from build123d import *

# Parameters (mm, degrees)
F1_DEPTH = 7.5


with BuildPart() as f1:
    # F0 (on Top) → F1 (new body)
    with BuildSketch(Plane.XY):
        with BuildLine():
            ThreePointArc((8.7951269587, 32.985141357), (9.3550716579, 31.5299513828), (9.8501945992, 30.0514490323))
            ThreePointArc((9.8501945992, 30.0514490323), (12.9209659931, 34.6103211779), (14, 40))
            ThreePointArc((14, 40), (-5.3896788221, 52.9209659931), (-9.8501945992, 30.0514490323))
            ThreePointArc((-9.8501945992, 30.0514490323), (-9.3550716579, 31.5299513828), (-8.7951269587, 32.985141357))
            ThreePointArc((-8.7951269587, 32.985141357), (-3.7160006536, 50.6185610674), (11.25, 40))
            ThreePointArc((11.25, 40), (10.6185610674, 36.2839993464), (8.7951269587, 32.985141357))
        make_face()
        with BuildLine():
            ThreePointArc((0, 26), (5.3254242297, 27.0524188833), (9.8501945992, 30.0514490323))
            ThreePointArc((9.8501945992, 30.0514490323), (9.3550716579, 31.5299513828), (8.7951269587, 32.985141357))
            ThreePointArc((8.7951269587, 32.985141357), (4.8808472762, 29.8639342017), (0, 28.75))
            Line((0, 28.75), (0, 26))
        make_face()
        with BuildLine():
            ThreePointArc((-9.8501945992, 30.0514490323), (-5.3254242297, 27.0524188833), (0, 26))
            Line((0, 26), (0, 28.75))
            ThreePointArc((0, 28.75), (-4.8808472762, 29.8639342017), (-8.7951269587, 32.985141357))
            ThreePointArc((-8.7951269587, 32.985141357), (-9.3550716579, 31.5299513828), (-9.8501945992, 30.0514490323))
        make_face()
        with BuildLine():
            ThreePointArc((0, 14), (5.4503386544, 12.8954956691), (10.040688359, 9.7562583646))
            ThreePointArc((10.040688359, 9.7562583646), (11.4358727735, 19.9178431142), (9.8501945992, 30.0514490323))
            ThreePointArc((9.8501945992, 30.0514490323), (5.3254242297, 27.0524188833), (0, 26))
            Line((0, 26), (0, 22.6483326405))
            Line((0, 22.6483326405), (5.2916659042, 22.6483326405))
            Line((5.2916659042, 22.6483326405), (5.2916659042, 14.8166660219))
            Line((5.2916659042, 14.8166660219), (0, 14.8166660219))
            Line((0, 14.8166660219), (0, 14))
        make_face()
        with BuildLine():
            ThreePointArc((-10.040688359, 9.7562583646), (-5.4503386544, 12.8954956691), (0, 14))
            Line((0, 14), (0, 14.8166660219))
            Line((0, 14.8166660219), (-5.7150004432, 14.8166660219))
            Line((-5.7150004432, 14.8166660219), (-5.7150004432, 22.6483326405))
            Line((-5.7150004432, 22.6483326405), (0, 22.6483326405))
            Line((0, 22.6483326405), (0, 26))
            ThreePointArc((0, 26), (-5.3254242297, 27.0524188833), (-9.8501945992, 30.0514490323))
            ThreePointArc((-9.8501945992, 30.0514490323), (-11.4358727735, 19.9178431142), (-10.040688359, 9.7562583646))
        make_face()
        with BuildLine():
            ThreePointArc((0, 11.25), (5.0410157742, 10.0573684413), (9.013218304, 6.7323395492))
            ThreePointArc((9.0132183039, 6.7323395492), (9.5611769089, 8.2326704367), (10.040688359, 9.7562583646))
            ThreePointArc((10.040688359, 9.7562583646), (5.4503386544, 12.8954956691), (0, 14))
            Line((0, 14), (0, 11.25))
        make_face()
        with BuildLine():
            ThreePointArc((9.013218304, 6.7323395492), (10.6761698638, 3.5470969877), (11.25, 0))
            Line((11.25, 0), (14, 0))
            ThreePointArc((14, 0), (12.9724638567, 5.2645210121), (10.040688359, 9.7562583646))
            ThreePointArc((10.040688359, 9.7562583646), (9.5611769089, 8.2326704367), (9.0132183039, 6.7323395492))
        make_face()
        with BuildLine():
            ThreePointArc((-9.013218304, 6.7323395492), (-5.0410157742, 10.0573684413), (0, 11.25))
            Line((0, 11.25), (0, 14))
            ThreePointArc((0, 14), (-5.4503386544, 12.8954956691), (-10.040688359, 9.7562583646))
            ThreePointArc((-10.040688359, 9.7562583646), (-9.5611769089, 8.2326704367), (-9.0132183039, 6.7323395492))
        make_face()
        with BuildLine():
            ThreePointArc((-11.25, 0), (-10.6761698638, 3.5470969877), (-9.013218304, 6.7323395492))
            ThreePointArc((-9.0132183039, 6.7323395492), (-9.5611769089, 8.2326704367), (-10.040688359, 9.7562583646))
            ThreePointArc((-10.040688359, 9.7562583646), (-12.9724638567, 5.2645210121), (-14, 0))
            Line((-14, 0), (-11.25, 0))
        make_face()
        with BuildLine():
            ThreePointArc((-10.040688359, -9.7562583646), (-9.5611769089, -8.2326704367), (-9.0132183039, -6.7323395492))
            ThreePointArc((-9.013218304, -6.7323395492), (-10.6761698638, -3.5470969877), (-11.25, 0))
            Line((-11.25, 0), (-14, 0))
            ThreePointArc((-14, 0), (-12.9724638567, -5.2645210121), (-10.040688359, -9.7562583646))
        make_face()
        with BuildLine():
            Line((14, 0), (11.25, 0))
            ThreePointArc((11.25, 0), (10.6761698638, -3.5470969877), (9.013218304, -6.7323395492))
            ThreePointArc((9.0132183039, -6.7323395492), (9.5611769089, -8.2326704367), (10.040688359, -9.7562583646))
            ThreePointArc((10.040688359, -9.7562583646), (12.9724638567, -5.2645210121), (14, 0))
        make_face()
        with BuildLine():
            ThreePointArc((10.040688359, -9.7562583646), (9.5611769089, -8.2326704367), (9.0132183039, -6.7323395492))
            ThreePointArc((9.013218304, -6.7323395492), (5.0410157742, -10.0573684413), (0, -11.25))
            Line((0, -11.25), (0, -14))
            ThreePointArc((0, -14), (5.4503386544, -12.8954956691), (10.040688359, -9.7562583646))
        make_face()
        with BuildLine():
            Line((0, -14), (0, -11.25))
            ThreePointArc((0, -11.25), (-5.0410157742, -10.0573684413), (-9.013218304, -6.7323395492))
            ThreePointArc((-9.0132183039, -6.7323395492), (-9.5611769089, -8.2326704367), (-10.040688359, -9.7562583646))
            ThreePointArc((-10.040688359, -9.7562583646), (-5.4503386544, -12.8954956691), (0, -14))
        make_face()
        with BuildLine():
            Line((0, -14.8166660219), (0, -14))
            ThreePointArc((0, -14), (-5.4503386544, -12.8954956691), (-10.040688359, -9.7562583646))
            ThreePointArc((-10.040688359, -9.7562583646), (-11.4358727735, -19.9178431142), (-9.8501945992, -30.0514490323))
            ThreePointArc((-9.8501945992, -30.0514490323), (-5.3254242297, -27.0524188833), (0, -26))
            Line((0, -26), (0, -22.6483326405))
            Line((0, -22.6483326405), (-5.7150004432, -22.6483326405))
            Line((-5.7150004432, -22.6483326405), (-5.7150004432, -14.8166660219))
            Line((-5.7150004432, -14.8166660219), (0, -14.8166660219))
        make_face()
        with BuildLine():
            ThreePointArc((9.8501945992, -30.0514490323), (11.4358727735, -19.9178431142), (10.040688359, -9.7562583646))
            ThreePointArc((10.040688359, -9.7562583646), (5.4503386544, -12.8954956691), (0, -14))
            Line((0, -14), (0, -14.8166660219))
            Line((0, -14.8166660219), (5.2916659042, -14.8166660219))
            Line((5.2916659042, -14.8166660219), (5.2916659042, -22.6483326405))
            Line((5.2916659042, -22.6483326405), (0, -22.6483326405))
            Line((0, -22.6483326405), (0, -26))
            ThreePointArc((0, -26), (5.3254242297, -27.0524188833), (9.8501945992, -30.0514490323))
        make_face()
        with BuildLine():
            ThreePointArc((14, -40), (12.9209659931, -34.6103211779), (9.8501945992, -30.0514490323))
            ThreePointArc((9.8501945992, -30.0514490323), (9.3550716579, -31.5299513828), (8.7951269587, -32.985141357))
            ThreePointArc((8.7951269587, -32.985141357), (10.6185610674, -36.2839993464), (11.25, -40))
            ThreePointArc((11.25, -40), (-3.7160006536, -50.6185610674), (-8.7951269587, -32.985141357))
            ThreePointArc((-8.7951269587, -32.985141357), (-9.3550716579, -31.5299513828), (-9.8501945992, -30.0514490323))
            ThreePointArc((-9.8501945992, -30.0514490323), (-5.3896788221, -52.9209659931), (14, -40))
        make_face()
        with BuildLine():
            Line((0, -28.75), (0, -26))
            ThreePointArc((0, -26), (-5.3254242297, -27.0524188833), (-9.8501945992, -30.0514490323))
            ThreePointArc((-9.8501945992, -30.0514490323), (-9.3550716579, -31.5299513828), (-8.7951269587, -32.985141357))
            ThreePointArc((-8.7951269587, -32.985141357), (-4.8808472762, -29.8639342017), (0, -28.75))
        make_face()
        with BuildLine():
            ThreePointArc((8.7951269587, -32.985141357), (9.3550716579, -31.5299513828), (9.8501945992, -30.0514490323))
            ThreePointArc((9.8501945992, -30.0514490323), (5.3254242297, -27.0524188833), (0, -26))
            Line((0, -26), (0, -28.75))
            ThreePointArc((0, -28.75), (4.8808472762, -29.8639342017), (8.7951269587, -32.985141357))
        make_face()
    extrude(amount=F1_DEPTH)


solid = f1.part
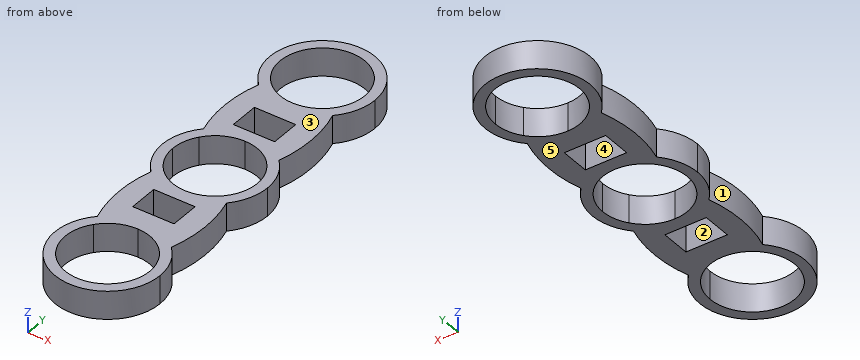
The listing builds one solid part. Answer for the finished solid, in the listing's coordinates (mm). Face numbers are marked on the shaded views. A direction names the side the tool comes from. Give positions to 0.01 mm unless a question says otherwise; leave off trailing zeros. Order: outer loops, then holes, each group sorted by start corner. A loop starts at its lowest first (then second) coordinate and runs counter-clockwise, first axis right, second up. Notation, with made-up numbers: (7.25, -35.5) -> (50.25, -35.5) arc R19 cw to (50.25, -20.5) -> close; hole circle Ø5 at (0, -35.5). An arc over 180 degrees is marked (long way). Put each result on its own line as item: value.
Item 1: For a pull along X with two mould halves and no side action, classify the marked faces 1, 2 and 3 as released by +X, released by -X, zero draft, split by the parting line, or undercut.
Established:
face 1: released by -X
face 2: undercut
face 3: zero draft
Item 2: Straight lines are drawn through the part: line 1 (X direction, y = -40, z = 5); line 2 (Y direction, x = 1.75, z = 5); line 3 (Y direction, x = -6.5, z = 3.5). For each, find the intervals that lie inside material, in ascending order.
Established:
line 1: x = -14 to -11.25, 11.25 to 14
line 2: y = -53.89 to -51.11, -28.89 to -22.65, -14.82 to -11.11, 11.11 to 14.82, 22.65 to 28.89, 51.11 to 53.89
line 3: y = -52.4 to -49.18, -30.82 to -9.18, 9.18 to 30.82, 49.18 to 52.4
Item 3: A cutting plane is placed at A-A on y = 2. Give the vertices of the cut face in (x, z), plus the area to 3 significant figures.
Established:
outline: (-13.86, 0) -> (-11.07, 0) -> (-11.07, 7.5) -> (-13.86, 7.5) -> close; (11.07, 0) -> (13.86, 0) -> (13.86, 7.5) -> (11.07, 7.5) -> close
area: 41.8 mm^2
Item 4: A cutting plane is placed at D-D on y = 18. Give the vertices of the cut face in (x, z) (3 decimals).
Established:
outline: (-11.402, 0) -> (-5.715, 0) -> (-5.715, 7.5) -> (-11.402, 7.5) -> close; (5.292, 0) -> (11.402, 0) -> (11.402, 7.5) -> (5.292, 7.5) -> close
Item 5: A cutting plane is placed at B-B on x = -2.5. Give the vertices of the cut face in (y, z), plus the area to 3 significant figures.
Established:
outline: (-53.77, 0) -> (-50.97, 0) -> (-50.97, 7.5) -> (-53.77, 7.5) -> close; (-29.03, 0) -> (-22.65, 0) -> (-22.65, 7.5) -> (-29.03, 7.5) -> close; (-14.82, 0) -> (-10.97, 0) -> (-10.97, 7.5) -> (-14.82, 7.5) -> close; (10.97, 0) -> (14.82, 0) -> (14.82, 7.5) -> (10.97, 7.5) -> close; (22.65, 0) -> (29.03, 0) -> (29.03, 7.5) -> (22.65, 7.5) -> close; (50.97, 0) -> (53.77, 0) -> (53.77, 7.5) -> (50.97, 7.5) -> close
area: 196 mm^2
Item 6: A cutting plane is placed at C-C on z = 6.5. Give the vertices of the cut face in (x, y) (3 decimals).
Established:
outline: (-10.041, -9.756) arc R35.292 ccw to (-9.85, -30.051) arc R14 ccw (long way) to (9.85, -30.051) arc R35.292 ccw to (10.041, -9.756) arc R14 ccw to (10.041, 9.756) arc R35.292 ccw to (9.85, 30.051) arc R14 ccw (long way) to (-9.85, 30.051) arc R35.292 ccw to (-10.041, 9.756) arc R14 ccw to start; hole circle Ø22.5 at (0, -40); hole circle Ø22.5 at (0, 0); hole circle Ø22.5 at (0, 40); hole (-5.715, -22.648) -> (5.292, -22.648) -> (5.292, -14.817) -> (-5.715, -14.817) -> close; hole (-5.715, 14.817) -> (5.292, 14.817) -> (5.292, 22.648) -> (-5.715, 22.648) -> close
Item 7: For the marked faces 4 and 5, determine the directions among +Z, -Z, +X, -X, +Y, -Y from which every point of the face is accessible in a straight line to the end or side of a thin tool.
Established:
face 4: +Z, -Z
face 5: -Z, +X, -X, +Y, -Y
Item 8: Given P1, Ø13.5, axis at x = 0, y = -40, coming from the +Z side; P2, Ø2, axis at x = -2.5, z = 4, coming from the +Y side; P3, Ø3, axis at x = 8, z = 1, coming from the -Y side; P4, Ø2, axis at y = 19, z = 3.5, coming from the +X side, each flat-ended and moving along its own axis, determine where each tip first touches the part or whether it passes through.
Established:
P1: passes through
P2: stops at y = 53.92
P3: stops at y = -52.4
P4: stops at x = 11.44
